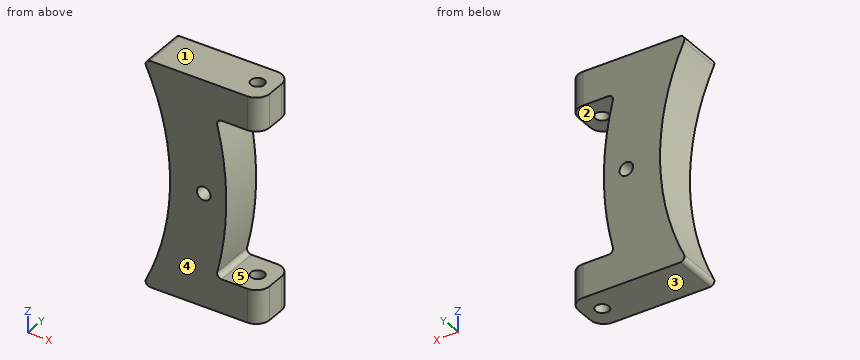
Autodesk Inventor part; units mm, degrees
ref_plane "YZ Plane" through (0, 0, 0) normal (1, 0, 0) x (0, 1, 0)
ref_plane "XZ Plane" through (0, 0, 0) normal (0, 1, 0) x (-1, 0, 0)
ref_plane "XY Plane" through (0, 0, 0) normal (0, 0, 1) x (1, 0, 0)
sketch "Sketch1" plane through (0, 0, 0) normal (0, 1, 0) x (-1, 0, 0)
  circle A0 centre (0, 0) radius 135
  circle A1 centre (0, 0) radius 110
  circle A2 centre (0, 0) radius 125
  circle A3 centre (-125, 0) radius 3
  circle A4 centre (-101.1271, -73.4732) radius 3
  circle A5 centre (-38.6271, -118.8821) radius 3
  circle A6 centre (38.6271, -118.8821) radius 3
  circle A7 centre (101.1271, -73.4732) radius 3
  circle A8 centre (125, 0) radius 3
  circle A9 centre (101.1271, 73.4732) radius 3
  circle A10 centre (38.6271, 118.8821) radius 3
  circle A11 centre (-38.6271, 118.8821) radius 3
  circle A12 centre (-101.1271, 73.4732) radius 3
  dimension "d68" = 250
  dimension "d0" = 270
  dimension "d1" = 220
  dimension "d74" = 6
  dimension "d77" = 360
extrude "Extrusion1" add sketch "Sketch1" along normal mid plane 20 contours A0 | A8 A2 A7 A6 A5 A4 A3 A12 A11 A10 A9
sketch "Sketch4" plane through (0, 10, 0) normal (0, 1, 0) x (1, 0, 0)
  circle A0 centre (0, 0) radius 50.125
  circle A1 centre (0, 0) radius 135
  circle A2 centre (0, 0) radius 110
  line L0 (125.3494, 50.125) -> (150.3494, 50.125)
  line L1 (150.3494, 50.125) -> (150.3494, 35.125)
  line L2 (150.3494, 35.125) -> (125.3494, 35.125)
  line L3 (125.3494, 35.125) -> (125.3494, 50.125)
  line L4 (150.3494, 70.125) -> (104.7795, 70.125)
  line L5 (104.7795, 70.125) -> (104.7795, 85.125)
  line L6 (104.7795, 85.125) -> (150.3494, 85.125)
  line L7 (150.3494, 85.125) -> (150.3494, 70.125)
  line L8 (103.1497, 60.125) -> (138.3886, 60.125) construction
  point P0 (130.3504, 35.125)
  point P1 (115.3581, 70.125)
  dimension "d21" = 100.25
  dimension "d22" = 25
  dimension "d23" = 15
  dimension "d24" = 20
  dimension "d25" = 15
  dimension "d57" = 10
extrude "Extrusion3" add sketch "Sketch4" against normal up to surface (20 mm away) contours L6 L7 L4 A1 | A1 L0 L1 L2
fillet "Fillet1" radius 6 4 edges at (150.3494, 10, -77.625) (150.3494, -10, -77.625) (150.3494, -10, -42.625) (150.3494, 10, -42.625)
fillet "Fillet2" radius 10 1 edges at (104.7795, 0, -85.125)
fillet "Fillet3" radius 2 1 edges at (130.3504, 0, -35.125)
sketch "Sketch5" plane through (150.3494, -4, -85.125) normal (0, 0, -1) x (-1, 0, 0)
  line L0 (0, 8) -> (0, 0)
  line L1 (40.9135, -6) -> (6, -6)
  point P0 (150.3494, 4)
  point P1 (8, 4)
  point P2 (0, 4)
  dimension "d38" = 8
  dimension "d39" = 10
hole "Hole2" at (142.3494, 0, -85.125) direction (0, 0, 1) diameter 6 depth 50 counterbore diameter 8.8 counterbore depth 5
mirror "Mirror1" about plane through (0, 0, 0) normal (1, 0, 0) of "Extrusion3", "Fillet1", "Fillet2", "Fillet3", "Hole2"
mirror "Mirror2" about plane through (0, 0, 0) normal (0, 0, 1) of "Extrusion3", "Fillet1", "Fillet2", "Fillet3", "Hole2"
sketch "Sketch7" plane through (0, 10, 0) normal (0, 1, 0) x (1, 0, 0)
  line L0 (0, 0) -> (0, -158.0698) construction
  point P0 (0, -127.5)
  dimension "d50" = 127.5
hole "Hole3" at (0, 10, 127.5) direction (0, -1, 0) diameter 5 end through all
sketch "Sketch10" plane through (0, 10, 0) normal (0, 1, 0) x (1, 0, 0)
  line L0 (144.3494, 50.125) -> (125.3494, 50.125)
  line L1 (144.3494, -50.125) -> (125.3494, -50.125)
  line L2 (174.7146, 50.125) -> (75.699, 50.125)
  line L3 (75.699, 50.125) -> (75.699, -50.125)
  line L4 (75.699, -50.125) -> (174.7146, -50.125)
  line L5 (174.7146, 145.3293) -> (-157.7861, 145.3293)
  line L6 (-157.7861, 145.3293) -> (-157.7861, -141.1771)
  line L7 (-157.7861, -141.1771) -> (174.7146, -141.1771)
  line L8 (174.7146, -141.1771) -> (174.7146, -50.125)
  line L9 (174.7146, 50.125) -> (174.7146, 145.3293)
  point P0 (0, 0)
extrude "Extrusion7" cut sketch "Sketch10" against normal through all
fillet "Fillet7" radius 2 2 edges at (97.9157, 0, -50.125) (97.9157, 0, 50.125)
properties part number "Cylinder 80-20 Spacer_1"
Could you check a few things on this model? Use its own coordinates, in mm. Face numbers are marked on the shaded views. A direction names the side the tool comes from. Give positions to 0.01 mm unless a question says otherwise; leave off trailing zeros. Order: outer loops, then holes, each group sorted by start corner. A loop starts at its lowest first (then second) coordinate and runs counter-clockwise, first axis right, second up.
1. Suppose I cut it at A-A (y = 0). Write out the boundary of the cut face in (x, z) (1 decimal).
Answers below:
outline: (99.3, -47.3) arc R2 ccw to (101.1, -50.1) - (139.3, -50.1) - (139.3, -35.1) - (132.9, -35.1) arc R2 cw to (131, -32.6) arc R135 ccw to (131, 32.6) arc R2 cw to (132.9, 35.1) - (139.3, 35.1) - (139.3, 50.1) - (101.1, 50.1) arc R2 ccw to (99.3, 47.3) arc R110 cw to start; (145.3, -50.1) - (150.3, -50.1) - (150.3, -35.1) - (145.3, -35.1) - close; (145.3, 35.1) - (150.3, 35.1) - (150.3, 50.1) - (145.3, 50.1) - close; hole circle Ø6 at (125, 0)
2. Suppose I cut it at C-C (x = 125). Write out the boundary of the cut face in (y, z) (3 decimals), plus the area to 4 significant figures.
Answers below:
outline: (-10, -50.125) - (10, -50.125) - (10, -3) - (-10, -3) - close; (-10, 3) - (10, 3) - (10, 50.125) - (-10, 50.125) - close
area: 1,885 mm2
3. Which directions (+Z, -Z, +X, -X, +Y, -Y) give clear straight access to the entire face, cutting with the end or side of a thin tool? Please do the marked faces 1 and 2.
Answers below:
face 1: +Z, +X, -X, +Y, -Y
face 2: +X, +Y, -Y
4. Suppose I cut it at B-B (z = 0). Write out the boundary of the cut face in (x, y).
Answers below:
outline: (110, -10) - (122, -10) - (122, 10) - (110, 10) - close; (128, -10) - (135, -10) - (135, 10) - (128, 10) - close
5. For pin 1 (3 mm diameter, centred on y = -1, z = 38, fed in from -X); pin 2 (4 mm diameter, centred on y = -2, z = 8.5, fed in from -X); pin 3 (12 mm diameter, centred on y = 7.5, z = -21.5, fed in from -X), each with a flat end and sliding along its axis, tell me the tip position at first contact or that it passes through.
Answers below:
pin 1: stops at x = 102.66
pin 2: stops at x = 109.5
pin 3: stops at x = 106.51
6. Suppose I cut it at D-D (y = -7.75). Write out the boundary of the cut face in (x, z) (1 decimal), plus the area to 3 significant figures.
Answers below:
outline: (99.3, -47.3) arc R2 ccw to (101.1, -50.1) - (149, -50.1) - (149, -35.1) - (132.9, -35.1) arc R2 cw to (131, -32.6) arc R135 ccw to (131, 32.6) arc R2 cw to (132.9, 35.1) - (149, 35.1) - (149, 50.1) - (101.1, 50.1) arc R2 ccw to (99.3, 47.3) arc R110 cw to start; hole circle Ø6 at (125, 0)
area: 3,180 mm2
7. Thinking about a two-plate mould opening in Z: for the marked faces 3, 4 and 5, which applies, +Z half, -Z half, draft (parallel to the pull), parting line (faces both ways), or undercut?
Answers below:
face 3: -Z half
face 4: draft
face 5: undercut
8. I need wall thicknesses on L1, parallel to Z at x = 140.5, y = -9 (3 decimals); L2, parallel to Z at x = 125, y = -4.5 (3 decimals); L3, parallel to X at y = -3.5, z = 20. Which ranges of each line are inside material? Lowest first, please.
Answers below:
L1: z = -50.125 to -35.125, 35.125 to 50.125
L2: z = -50.125 to -3, 3 to 50.125
L3: x = 108.17 to 133.51
